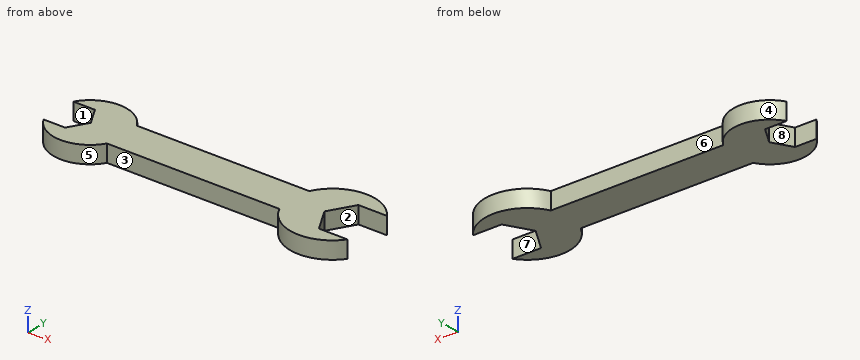
```python
from build123d import *

# Parameters (mm, degrees)
F1_DEPTH = 6


with BuildPart() as f1:
    # F0 (on Top) → F1 (new body)
    with BuildSketch(Plane.XY):
        with BuildLine():
            Line((-49.6510066098, 0), (-49.6510066098, 6.5))
            Line((-49.6510066098, 6.5), (-38.8557657197, 6.5))
            ThreePointArc((-38.8557657197, 6.5), (-49.8825512893, 12.8), (-60.909336859, 6.5))
            Line((-60.909336859, 6.5), (-53.4037833596, 6.5))
            Line((-53.4037833596, 6.5), (-49.6510066098, 0))
        make_face()
        with BuildLine():
            Line((-38.8557657197, 6.5), (-49.6510066098, 6.5))
            Line((-49.6510066098, 6.5), (-49.6510066098, 0))
            Line((-49.6510066098, 0), (-49.6510066098, -6.5))
            Line((-49.6510066098, -6.5), (-38.8557657197, -6.5))
            ThreePointArc((-38.8557657197, -6.5), (-37.5338093435, -3.3687642176), (-37.0825512893, 0))
            ThreePointArc((-37.0825512893, 0), (-37.5338093435, 3.3687642176), (-38.8557657197, 6.5))
        make_face()
        with BuildLine():
            Line((-49.6510066098, -6.5), (-49.6510066098, 0))
            Line((-49.6510066098, 0), (-53.4037833596, -6.5))
            Line((-53.4037833596, -6.5), (-60.909336859, -6.5))
            ThreePointArc((-60.909336859, -6.5), (-49.8825512893, -12.8), (-38.8557657197, -6.5))
            Line((-38.8557657197, -6.5), (-49.6510066098, -6.5))
        make_face()
        with BuildLine():
            Line((21.0090092811, 6.5), (-38.8557657197, 6.5))
            ThreePointArc((-38.8557657197, 6.5), (-37.5338093435, 3.3687642176), (-37.0825512893, 0))
            ThreePointArc((-37.0825512893, 0), (-37.5338093435, -3.3687642176), (-38.8557657197, -6.5))
            Line((-38.8557657197, -6.5), (21.0090092811, -6.5))
            ThreePointArc((21.0090092811, -6.5), (19.5052493512, 0), (21.0090092811, 6.5))
        make_face()
        with BuildLine():
            ThreePointArc((46.3501652911, 8.6), (33.0829756422, 14.74944226), (21.0090092811, 6.5))
            Line((21.0090092811, 6.5), (31.454528346, 6.5))
            Line((31.454528346, 6.5), (31.454528346, 0))
            Line((31.454528346, 0), (36.419740661, 8.6))
            Line((36.419740661, 8.6), (46.3501652911, 8.6))
        make_face()
        with BuildLine():
            Line((31.454528346, 6.5), (21.0090092811, 6.5))
            ThreePointArc((21.0090092811, 6.5), (19.5052493512, 0), (21.0090092811, -6.5))
            Line((21.0090092811, -6.5), (31.454528346, -6.5))
            Line((31.454528346, -6.5), (31.454528346, 0))
            Line((31.454528346, 0), (31.454528346, 6.5))
        make_face()
        with BuildLine():
            Line((31.454528346, -6.5), (21.0090092811, -6.5))
            ThreePointArc((21.0090092811, -6.5), (33.0829756422, -14.74944226), (46.3501652911, -8.6))
            Line((46.3501652911, -8.6), (36.419740661, -8.6))
            Line((36.419740661, -8.6), (31.454528346, 0))
            Line((31.454528346, 0), (31.454528346, -6.5))
        make_face()
    extrude(amount=F1_DEPTH)


solid = f1.part
```
For this review, take the finished solid that the model builds, in its own axes (mm). Face numbers are marked on the shaded views. A direction names the side the tool comes from. Give positions to 0.01 mm unless a question says otherwise; leave off trailing zeros. Write each loop counter-clockwise with the first axis right and the second up, starting at its lowest first coordinate (ties: lowest second). Pieces come first, ordered by that corner, then holes.
Item 1: Machinability: for the marked faces 1, 2, 3 and 4, which of the approach directions +Z, -Z, +X, -X, +Y, -Y give a long, thin tool a straight path to every point of the face, cutting with its end or side? Answer none if there is none.
Item 2: Insertion check: P1, Ø1, axis at y = -4.5, z = 2.5, coming from the +X side; P2, Ø3, axis at y = -6.5, z = 4.5, coming from the +X side; P3, Ø3, axis at x = -16, z = 3.5, coming from the -Y side. Each pin has a flat end and moves straight along its axis. Give the tip position at first contact, or say it passes through.
Item 3: Wall thickness on probe 1 along Y at (x, z) = (-12.5, 4.5); probe 2 along X at (y, z) = (10.5, 2.9) (1 decimal); probe 3 along Y at (x, z) = (32, 3.45): over which ranges is each line inside the solid? List them lowest first.
Item 4: Take a section at B-B (y = 10.75). Give the boundary of the cut face in (x, z), and give its area (3 significant figures).
Item 5: Take a section at A-A (x = -51). Give the boundary of the cut face in (y, z).
Item 6: The part is to be moulded in two halves that separate along X. For the marked faces 5, 6, 7 and 8, say which applies: +X half, -X half, draft (parallel to the pull), parting line (faces both ways), or undercut.
Item 7: Take a section at C-C (z = 2.7). Give the boundary of the cut face in (x, y), and give its area (3 significant figures).
Item 8: Take a section at D-D (x = -37). Give the boundary of the cut face in (y, z), and give its area (3 significant figures).
Established:
1. face 1: +Z, -Z, -X
1. face 2: +Z, -Z, +X
1. face 3: +Z, -Z, -Y
1. face 4: +Z, -Z, +Y
2. P1: stops at x = 34.34
2. P2: stops at x = 36.07
2. P3: stops at y = -6.5
3. probe 1: y = -6.5 to 6.5
3. probe 2: x = -57.2 to -42.6, 23.9 to 44.7
3. probe 3: y = -14.62 to -0.94, 0.94 to 14.62
4. outline: (-56.83, 0) - (-42.93, 0) - (-42.93, 6) - (-56.83, 6) - close; (24.13, 0) - (44.48, 0) - (44.48, 6) - (24.13, 6) - close
4. area: 205 mm2
5. outline: (-12.75, 0) - (-2.34, 0) - (-2.34, 6) - (-12.75, 6) - close; (2.34, 0) - (12.75, 0) - (12.75, 6) - (2.34, 6) - close
6. face 5: undercut
6. face 6: undercut
6. face 7: draft
6. face 8: -X half
7. outline: (-60.91, -6.5) arc R12.8 ccw to (-38.86, -6.5) - (21.01, -6.5) arc R14.8 ccw to (46.35, -8.6) - (36.42, -8.6) - (31.45, 0) - (36.42, 8.6) - (46.35, 8.6) arc R14.8 ccw to (21.01, 6.5) - (-38.86, 6.5) arc R12.8 ccw to (-60.91, 6.5) - (-53.4, 6.5) - (-49.65, 0) - (-53.4, -6.5) - close
7. area: 1,570 mm2
8. outline: (-6.5, 0) - (6.5, 0) - (6.5, 6) - (-6.5, 6) - close
8. area: 78.0 mm2
